```python
from build123d import *

# Parameters (mm, degrees)
SKETCH_W        = 12.8
SKETCH_H        = 9.8
PAD_DEPTH       = 10
POCKET_DEPTH    = 5
SKETCH002_W     = 15
SKETCH002_H     = 12
PAD001_DEPTH    = 1
CHAMFER_SIZE    = 1
SKETCH003_W     = 3
SKETCH003_H     = 6
POCKET001_DEPTH = 9


with BuildPart() as part:
    # Sketch → Pad (new body)
    with BuildSketch(Plane.XY):
        Rectangle(SKETCH_W, SKETCH_H)
    extrude(amount=PAD_DEPTH)

    # Sketch001 (on Face6 of Pad) → Pocket (cut)
    with BuildSketch(Plane.XY.offset(10)):
        Polygon((-3.99861, 2.2628), (-3.99861, 1.7628), (-2.99861, 1.7628), (-2.99861, -2.2372), (-2.49861, -2.2372), (-2.49861, 1.7628), (-1.49861, 1.7628), (-1.49861, 2.2628), align=None)
        with BuildLine():
            ThreePointArc((1.047539, 1.197216), (-0.867234, 1.635805), (-0.050275, -0.150615))
            ThreePointArc((-0.630407, -1.305236), (0.670164, -1.235647), (-0.050275, -0.150615))
            Line((-1.130407, -1.322386), (-0.630407, -1.305236))
            ThreePointArc((-1.130407, -1.322386), (0.939152, -1.657302), (0.175897, 0.295308))
            ThreePointArc((0.547539, 1.20235), (-0.580104, 1.134721), (0.175897, 0.295308))
            Line((0.547539, 1.20235), (1.047539, 1.197216))
        make_face()
        with BuildLine():
            ThreePointArc((4, 2.186018), (1.813982, 0), (4, -2.186018))
            Line((4, -1.5), (4, -2.186018))
            ThreePointArc((4, 1.5), (2.5, 0), (4, -1.5))
            Line((4, 2.186018), (4, 1.5))
        make_face()
    extrude(amount=-POCKET_DEPTH, mode=Mode.SUBTRACT)

    # Sketch002 (on Face4 of Pocket) → Pad001 (join)
    with BuildSketch(Plane(origin=(0, 0, 0), x_dir=(1, 0, 0), z_dir=(0, 0, -1))):
        Rectangle(SKETCH002_W, SKETCH002_H)
    extrude(amount=PAD001_DEPTH)

    # Chamfer
    chamfer_edges = [part.edges().sort_by_distance(p)[0] for p in [
        (6.4, -4.9, 5),
        (-6.4, -4.9, 5),
        (0, -4.9, 10),
        (-6.4, 0, 10),
        (0, 4.9, 10),
        (6.4, 0, 10),
        (6.4, 4.9, 5),
        (-6.4, 4.9, 5),
    ]]
    chamfer(chamfer_edges, length=CHAMFER_SIZE)

    # Sketch003 (on Face22 of Chamfer) → Pocket001 (cut)
    with BuildSketch(Plane(origin=(0, 0, -1), x_dir=(1, 0, 0), z_dir=(0, 0, -1))):
        with Locations((-3.162799, 0)):
            Rectangle(SKETCH003_W, SKETCH003_H)
        with Locations((3.322114, 0)):
            Rectangle(SKETCH003_W, SKETCH003_H)
    extrude(amount=-POCKET001_DEPTH, mode=Mode.SUBTRACT)


solid = part.part
```
The model under review builds one solid part; all positions refer to its coordinate system, in mm. A direction names the side the tool comes from. Give positions to 0.01 mm unless a question says otherwise; leave off trailing zeros. Write each loop counter-clockwise with the first axis right and the second up, starting at its lowest first coordinate (ties: lowest second). Pieces come first, ordered by that corner, then holes. Notation, with made-up numbers: (-32.5, 42) -> (-8.5, 42) arc R18 cw to (-8.5, 54) -> close; hole circle Ø2 at (-30.5, -25.75). An arc over 180 degrees is marked (long way). Answer in a Markdown table with one row per item.
1) Mouldability with a two-part tool opening along X and no side actions: class faces 6 (the flat face through (5.9, -4.4, 4.4)), 7 (the flat face through (-5.7, -4.2, 9.4)), 8 (the flat face through (-3.2, 0, 8)), 9 (the flat face through (-3, -3, 3)) as +X half, -X half, draft (parallel to the pull), parting line (faces both ways), or undercut.
Worked answers:
| item | result |
|---|---|
| face 6 | +X half |
| face 7 | -X half |
| face 8 | undercut |
| face 9 | undercut |
2) Add section C-C on y = 3.5. State the section outline as (x, z) points, plus the area to 3 significant figures.
Worked answers:
| item | result |
|---|---|
| outline | (-7.5, -1) -> (7.5, -1) -> (7.5, 0) -> (6.4, 0) -> (6.4, 9) -> (5.4, 10) -> (-5.4, 10) -> (-6.4, 9) -> (-6.4, 0) -> (-7.5, 0) -> close |
| area | 142 mm² |
3) Add section D-D on y = -1. Count the separate pieces of the cut face and the enclosed holes in it, plus the area to 3 significant figures.
Worked answers:
| item | result |
|---|---|
| separate pieces | 3 |
| enclosed holes | 0 |
| area | 83.0 mm² |
4) Add section A-A on x = -3.75. State the section outline as (y, z) points, plus the area to 3 significant figures.
Worked answers:
| item | result |
|---|---|
| outline | (-6, -1) -> (-3, -1) -> (-3, 8) -> (1.76, 8) -> (1.76, 10) -> (-3.9, 10) -> (-4.9, 9) -> (-4.9, 0) -> (-6, 0) -> close; (2.26, 8) -> (3, 8) -> (3, -1) -> (6, -1) -> (6, 0) -> (4.9, 0) -> (4.9, 9) -> (3.9, 10) -> (2.26, 10) -> close |
| area | 54.0 mm² |
5) For L1, parallel to X at y = -2.5, z = 2.25; L2, parallel to Y at x = -3.75, z = 1.25; L3, parallel to Y at x = 3, z = 8.5, list the stretches that pass through material, from the lowest coordinate up. Write a range as [from, to].
Worked answers:
| item | result |
|---|---|
| L1 | [-6.4, -4.66], [-1.66, 1.82], [4.82, 6.4] |
| L2 | [-4.9, -3], [3, 4.9] |
| L3 | [-4.9, -1.94], [-1.12, 1.12], [1.94, 4.9] |
6) Add section B-B on z = 3.5. State the section outline as (x, y) points, plus the area to 3 significant figures.
Worked answers:
| item | result |
|---|---|
| outline | (-6.4, -3.9) -> (-5.4, -4.9) -> (5.4, -4.9) -> (6.4, -3.9) -> (6.4, 3.9) -> (5.4, 4.9) -> (-5.4, 4.9) -> (-6.4, 3.9) -> close; hole (-4.66, -3) -> (-1.66, -3) -> (-1.66, 3) -> (-4.66, 3) -> close; hole (1.82, -3) -> (4.82, -3) -> (4.82, 3) -> (1.82, 3) -> close |
| area | 87.4 mm² |
7) Clearance check with flat-ended pins moving along their axes: P1, Ø0.6, axis at y = 2, z = 8, coming from the -X side; P2, Ø2, axis at x = -5.5, z = 7, coming from the +Y side; P3, Ø1.5, axis at y = 2.5, z = 6, coming from the +X side; P4, Ø4, axis at x = -3, z = 1.5, coming from the -Y side. State where each tip first meets the part, or that it passes through.
Worked answers:
| item | result |
|---|---|
| P1 | x = -6.4 |
| P2 | y = 4.9 |
| P3 | x = 6.4 |
| P4 | y = -6 |
8) Tool access review of faces 1 (the flat face through (-5.9, -0.1, 9.5)), 2 (the flat face through (0, -4.9, 4)), 3 (the flat face through (0, 4.9, 4)), 4 (the flat face through (3, 3, 3)), 5 (the flat face through (-2, 1.763, 9)): name each direction out of +Z, -Z, +X, -X, +Y, -Y from which nothing blocks a thin tool from reaching the whole face with its end or side.
Worked answers:
| item | result |
|---|---|
| face 1 | +Z, -X, +Y, -Y |
| face 2 | +Z, +X, -X, -Y |
| face 3 | +Z, +X, -X, +Y |
| face 4 | -Z |
| face 5 | +Z |
